Could you check a few things on this model? Use its own coordinates, in mm. Round coordinates to 2 decimals unless told otherwise and drop trailing zeros. Loops run counter-clockwise (first coordinate to the right, second up) from the corner with the lowest first, then second, coordinate; pieces in that order, holes last. Notation, with made-up numbers: (-11, 55) -> (29, 55) arc R9 cw to (29, 70) -> close; hole circle Ø10 at (8, 8). An arc over 180 degrees is marked (long way). Use CSV: the item, a comma, the result in double quotes. Start each with the question number.
```python
from build123d import *

# Parameters (mm, degrees)
F0_W     = 3
F0_H     = 16.165595
F0_H_2   = 12.856834
F1_DEPTH = 3


with BuildPart() as f1:
    # F0 (on Right) → F1 (new body)
    with BuildSketch(Plane.YZ):
        Polygon((101.258113, 32.087279), (-25.741887, 61.851164), (-25.741887, -141.348836), (101.258113, -120.312721), align=None)
        with Locations((-21.8319, -82.466038)):
            Rectangle(F0_W, F0_H, mode=Mode.SUBTRACT)
        with Locations((-11.68815, -82.466038)):
            Rectangle(F0_W, F0_H, mode=Mode.SUBTRACT)
        with Locations((-21.991294, 7.635576)):
            Rectangle(F0_W, F0_H_2, mode=Mode.SUBTRACT)
        with Locations((-11.853894, 7.635576)):
            Rectangle(F0_W, F0_H_2, mode=Mode.SUBTRACT)
    extrude(amount=F1_DEPTH)


solid = f1.part
```
1. Suppose I cut it at B-B (y = 57.5). List the corners of the cut face in (x, z) for me, then the cut area to 3 significant figures.
2. Will these pins go through, and if not, where does the flat tip stop? pin 1 (1.5 mm diameter, centred on x = 1.5, y = -12, fed in from -Z); pin 2 (1.5 mm diameter, centred on x = 1, y = -11.5, fed in from +Z).
3. Suppose I cut it at C-C (y = 43.5). List the corners of the cut face in (x, z) for me, then the cut area to 3 significant figures.
4. Suppose I cut it at A-A (x = 2). List the corners of the cut face in (y, z) for me.
5. If I drill on L1, parallel to Y at x = 1.35, z = -84; L2, parallel to Z at x = 2.1, y = -12; L3, parallel to Z at x = 2.5, y = 43.5, over which ranges is the centre line in solid material (lowest first)?
Geometry check:
1,outline,"(0, -127.56) -> (3, -127.56) -> (3, 42.34) -> (0, 42.34) -> close"
1,area,"510 mm²"
2,pin 1,"stops at z = -139.2"
2,pin 2,"stops at z = 58.69"
3,outline,"(0, -129.88) -> (3, -129.88) -> (3, 45.62) -> (0, 45.62) -> close"
3,area,"527 mm²"
4,outline,"(-25.74, -141.35) -> (101.26, -120.31) -> (101.26, 32.09) -> (-25.74, 61.85) -> close; hole (-23.49, 1.21) -> (-20.49, 1.21) -> (-20.49, 14.06) -> (-23.49, 14.06) -> close; hole (-23.33, -90.55) -> (-20.33, -90.55) -> (-20.33, -74.38) -> (-23.33, -74.38) -> close; hole (-13.35, 1.21) -> (-10.35, 1.21) -> (-10.35, 14.06) -> (-13.35, 14.06) -> close; hole (-13.19, -90.55) -> (-10.19, -90.55) -> (-10.19, -74.38) -> (-13.19, -74.38) -> close"
5,L1,"y = -25.74 to -23.33, -20.33 to -13.19, -10.19 to 101.26"
5,L2,"z = -139.07 to -90.55, -74.38 to 1.21, 14.06 to 58.63"
5,L3,"z = -129.88 to 45.62"
